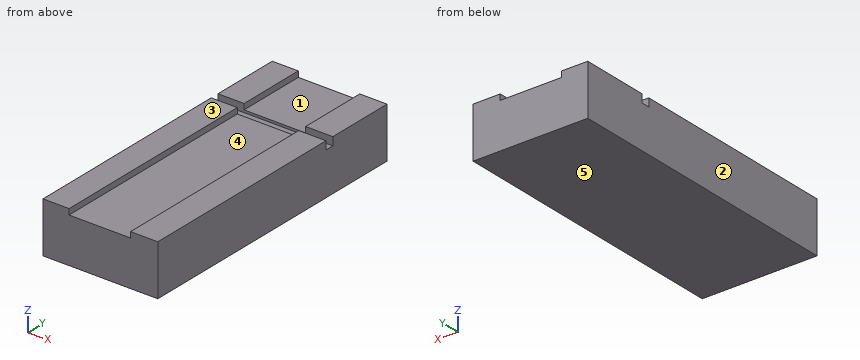
```python
from build123d import *

# Parameters (mm, degrees)
F0_W     = 1.6141478449
F0_H     = 17.9891760959
F0_W_2   = 3.81
F0_W_3   = 1.6878521551
F1_DEPTH = 3.1496
F2_START = 2.794
F2_DEPTH = 2.0828
F3_W     = 8.6175605327
F3_H     = 0.5334
F3_W_2   = 1.6141478449
F4_DEPTH = 0.508


with BuildPart() as f1:
    # F0 (on Top) → F1 (new body)
    with BuildSketch(Plane.XY):
        with Locations((-3.3795093424, -0.3924611956)):
            Rectangle(F0_W, F0_H)
        with Locations((-0.66743542, -0.3924611956)):
            Rectangle(F0_W_2, F0_H)
        with Locations((2.0814906576, -0.3924611956)):
            Rectangle(F0_W_3, F0_H)
    extrude(amount=F1_DEPTH)

    # F0 (on Top) → F2 (cut)
    with BuildSketch(Plane.XY.offset(F2_START)):
        with Locations((-0.66743542, -0.3924611956)):
            Rectangle(F0_W_2, F0_H)
    extrude(amount=F2_DEPTH, mode=Mode.SUBTRACT)

    # F3 (on face) → F4 (cut)
    with BuildSketch(Plane.XY.offset(3.1496)):
        with Locations((1.7363448463, 4.0817503403)):
            Rectangle(F3_W, F3_H)
        with Locations((-3.3795093424, 4.0817503403)):
            Rectangle(F3_W_2, F3_H)
    extrude(amount=-F4_DEPTH, mode=Mode.SUBTRACT)


solid = f1.part
```
Part model, mm, in its own coordinate system. Face numbers are marked on the shaded views. A direction names the side the tool comes from. Round coordinates to 2 decimals unless told otherwise and drop trailing zeros. Order: outer loops, then holes, each group sorted by start corner. A loop starts at its lowest first (then second) coordinate and runs counter-clockwise, first axis right, second up. Notation, with made-up numbers: M 30,89.5 L 82,89.5 A14 cw 82,95.5 Z; hole C 46,2.25 d2. An arc over 180 degrees is marked long. Answer in a Markdown table with one row per item. Add a question column.
Q1. Mould opens along X. For the marked faces 1, 2 and 3 say: +X half, -X half, draft (parallel to the pull), parting line (faces both ways), or undercut.
Q2. Wall check: L1, parallel to Y at x = 0.75, z = 2.75; L2, parallel to X at y = -1.5, z = 2.85; L3, parallel to Z at x = -1, y = 6.25. Give the ranges that are in metal, low to high. Write a range as from..to.
Q3. Cut at B-B on y = -6. Give the cut face in (x, z).
Q4. Pin check, flat tip, straight feed: pin 1 (0.6 mm diameter, centred on x = 0, y = 4, fed in from +Z). Stop position of the tip, or through.
Q5. Cut at A-A on x = -0.75. Give the cut face in (y, z), and give its area (3 significant figures).
Q6. 3-axis set-ups, long thin cutter, end or side, ignore diameter. For the marked faces 4 and 5: which of +Z, -Z, +X, -X, +Y, -Y reach the whole face in a straight line?
Established:
| question | item | result |
|---|---|---|
| 1 | face 1 | undercut |
| 1 | face 2 | -X half |
| 1 | face 3 | draft |
| 2 | L1 | y = -9.39..3.82, 4.35..8.6 |
| 2 | L2 | x = -4.19..-2.57, 1.24..2.93 |
| 2 | L3 | z = 0..2.79 |
| 3 | outline | M -4.19,0 L 2.93,0 L 2.93,3.15 L 1.24,3.15 L 1.24,2.79 L -2.57,2.79 L -2.57,3.15 L -4.19,3.15 Z |
| 4 | pin 1 | stops at z = 2.79 |
| 5 | outline | M -9.39,0 L 8.6,0 L 8.6,2.79 L 4.35,2.79 L 4.35,2.64 L 3.82,2.64 L 3.82,2.79 L -9.39,2.79 Z |
| 5 | area | 50.2 mm2 |
| 6 | face 4 | +Z, +Y, -Y |
| 6 | face 5 | -Z, +X, -X, +Y, -Y |
